```python
from build123d import *

# Parameters (mm, degrees)
SKETCH_1_R      = 38
EXTRUDE_1_DEPTH = 10
FILLET_1_R      = 130


with BuildPart() as part:
    # 草图1 → 凸台-拉伸1 (new body)
    with BuildSketch(Plane(origin=(0, 0, 0), x_dir=(1, 0, 0), z_dir=(0, 1, 0))):
        with Locations(Location((0, 0, 0), (0, 0, 270))):
            Circle(SKETCH_1_R)
    extrude(amount=EXTRUDE_1_DEPTH)

    # 草图3 → 旋转1 (revolve)
    with BuildSketch(Plane.XY, mode=Mode.PRIVATE) as revolve_1_sk:
        Polygon((0, 130), (11, 130), (11, 40), (38, 10), (0, 10), align=None)
    revolve(revolve_1_sk.sketch.rotate(Axis((0, 0, 0), (0, 1, 0)), 90), axis=Axis((0, 0, 0), (0, 1, 0)))

    # 圆角1
    # the kernel refuses this fillet: 130 mm, written as the material it adds along each edge
    with BuildSketch(Plane(origin=(0, 40, 0), x_dir=(0, 0, -1), z_dir=(1, 0, 0))) as fillet_1_piece_1:
        with BuildLine():
            CenterArc((141, 49.315824398), FILLET_1_R, 180, 37.598305078)
            Line((11, 49.315824398), (8.4, 49.315824398))
            Line((8.4, 49.315824398), (8.4, 0))
            Line((8.4, 0), (9.06743522, -1.739308302))
            ThreePointArc((9.06743522, -1.739308302), (22.56743522, -16.739308302), (35.94, -31.586316488))
            Line((35.94, -31.586316488), (38, -30))
        make_face()
    revolve(axis=Axis((0, 40, 0), (0, 1, 0)))


solid = part.part
```
Geometry check sheet. Reference: the model listing, model coordinates, mm. A direction names the side the tool comes from. Coordinates: 2 decimals unless noted, no trailing zeros. Order: outer loops, then holes, each group sorted by start corner. A loop starts at its lowest first (then second) coordinate and runs counter-clockwise, first axis right, second up.
Item 1: Section check D-D (y = 18). Enter the section's corners in (x, z).
Item 2: Depth check by flat-ended pin: pin 1 (1 mm diameter, centred on x = 1, y = 91.5, fed in from +Z); pin 2 (2 mm diameter, centred on y = 13, z = -19, fed in from +X); pin 3 (3 mm diameter, centred on x = -0.5, z = -26, fed in from -Y); pin 4 (5 mm diameter, centred on x = 6.5, y = 82, fed in from +Z). Enter the tip coordinate at first touch or a pass-through.
Item 3: Tool access check on faces 1 (the cylindrical face through (-23.122, 4.93, -30.156)), 2 (the cylindrical face through (10.74, 109.37, 2.38)). Record the directions out of +Z, -Z, +X, -X, +Y, -Y that give a thin tool (end or side, any length) a straight path to the whole face; none if there is none.
Item 4: Section check A-A (z = 0). Enter the section's corners in (x, y), plus the area to 3 significant figures.
Item 5: Section check B-B (x = 0). Enter the section's corners in (y, z), plus the area to 3 significant figures.
Item 6: Section check C-C (y = 109). Enter the section's corners in (x, z), plus the area to 3 significant figures.
Item 7: Scan lines: line 1 along Z through (x, y) = (-34, 8); line 2 along Z through (x, y) = (5, 36); line 3 along Y through (x, z) = (-23.5, 15.5). Record each from-to range of solid material in increasing order.
Check sheet entries:
1. outline: circle Ø64.62 at (0, 0)
2. pin 1: stops at z = 10.99
2. pin 2: stops at x = 31.34
2. pin 3: stops at y = 0
2. pin 4: stops at z = 10.48
3. face 1: +Y, -Y
3. face 2: +Y
4. outline: (-38, 0) - (38, 0) - (38, 10) arc R130 cw to (11, 89.32) - (11, 130) - (-11, 130) - (-11, 89.32) arc R130 cw to (-38, 10) - close
4. area: 4,760 mm2
5. outline: (0, -38) - (10, -38) arc R130 cw to (89.32, -11) - (130, -11) - (130, 11) - (89.32, 11) arc R130 cw to (10, 38) - (0, 38) - close
5. area: 4,760 mm2
6. outline: circle Ø22 at (0, 0)
6. area: 380 mm2
7. line 1: z = -16.97 to 16.97
7. line 2: z = -21.87 to 21.87
7. line 3: y = 0 to 24.78
